Here's how the part is built. I have some questions about the finished solid (model axes, mm). Coordinates: 2 decimals unless noted, no trailing zeros. Loops run counter-clockwise (first coordinate to the right, second up) from the corner with the lowest first, then second, coordinate; pieces in that order, holes last.
from build123d import *

# Parameters (mm, degrees)
SKETCH1_W                 = 12.7
SKETCH1_H                 = 444.5
EXTRUDE1_DEPTH            = 292.1
EXTRUDE1_DEPTH_BACK       = 292.1
CUT_EXTRUDE1_REACH        = 14.7
CUT_EXTRUDE2_REACH        = 14.7
SKETCH5_W                 = 127
SKETCH5_H                 = 43.65625
FILLET2_R                 = 6.35
M6X1_0_TAPPED_HOLE1_D     = 5
M6X1_0_TAPPED_HOLE1_DEPTH = 12.7
SKETCH11_W                = 292.1
SKETCH11_H                = 14.2875
CUT_EXTRUDE3_DEPTH        = 13.7
FILLET3_R                 = 3.175
CUT_EXTRUDE7_DEPTH        = 1
CUT_EXTRUDE7_DEPTH_BACK   = 445.5
CUT_EXTRUDE8_REACH        = 14.7
M6X1_0_TAPPED_HOLE2_D     = 5
M6X1_0_TAPPED_HOLE2_DEPTH = 12.7
M6_CLEARANCE_HOLE1_D      = 6.4
M6_CLEARANCE_HOLE1_DEPTH  = 12.7
CUT_EXTRUDE9_DEPTH        = 13.7
CUT_EXTRUDE10_DEPTH       = 13.7


with BuildPart() as part:
    # Sketch1 → Extrude1 (new body, two sides)
    with BuildSketch(Plane.XY) as extrude1_sk:
        Rectangle(SKETCH1_W, SKETCH1_H)
    extrude(amount=EXTRUDE1_DEPTH)
    extrude(extrude1_sk.sketch, amount=-EXTRUDE1_DEPTH_BACK)

    # Sketch4 → Cut-Extrude1 (cut, up to next)
    with BuildSketch(Plane(origin=(6.35, 0, 0), x_dir=(0, 0, -1), z_dir=(1, 0, 0)), mode=Mode.PRIVATE) as cut_extrude1_sk1:
        Polygon((203.2, 127.79375), (241.3, 127.79375), (241.3, 178.59375), (-241.3, 178.59375), (-241.3, 127.79375), (-203.2, 127.79375), (-203.2, -54.76875), (-241.3, -54.76875), (-241.3, -105.56875), (241.3, -105.56875), (241.3, -54.76875), (203.2, -54.76875), align=None)
    cut_extrude1_tool1 = extrude(cut_extrude1_sk1.sketch, amount=-CUT_EXTRUDE1_REACH, mode=Mode.PRIVATE) & part.part
    add(cut_extrude1_tool1.solids().sort_by_distance((6.35, 36.5125, 0))[0], mode=Mode.SUBTRACT)

    # Sketch5 → Cut-Extrude2 (cut, up to next)
    with BuildSketch(Plane(origin=(6.35, 0, 0), x_dir=(0, 0, -1), z_dir=(1, 0, 0)), mode=Mode.PRIVATE) as cut_extrude2_sk1:
        with Locations((0, 200.421875)):
            Rectangle(SKETCH5_W, SKETCH5_H)
    cut_extrude2_tool1 = extrude(cut_extrude2_sk1.sketch, amount=-CUT_EXTRUDE2_REACH, mode=Mode.PRIVATE) & part.part
    add(cut_extrude2_tool1.solids().sort_by_distance((6.35, 200.421875, 0))[0], mode=Mode.SUBTRACT)

    # Fillet2
    fillet2_edges = [part.edges().sort_by_distance(p)[0] for p in [
        (0, 127.79375, -203.2),
        (0, -54.76875, -203.2),
        (0, -54.76875, -241.3),
        (0, -105.56875, -241.3),
        (0, -105.56875, 241.3),
        (0, -54.76875, 241.3),
        (0, -54.76875, 203.2),
        (0, 127.79375, 203.2),
        (0, 127.79375, 241.3),
        (0, 178.59375, 241.3),
        (0, 178.59375, -241.3),
        (0, 127.79375, -241.3),
    ]]
    fillet(fillet2_edges, radius=FILLET2_R)

    # M6x1.0 Tapped Hole1
    with Locations(Plane(origin=(6.35, 0, 0), x_dir=(0, 0, -1), z_dir=(1, 0, 0))):
        with Locations((101.6, 204.7875), (-101.6, 204.7875), (101.6, -132.23875), (-101.6, -132.23875)):
            Hole(M6X1_0_TAPPED_HOLE1_D / 2, depth=M6X1_0_TAPPED_HOLE1_DEPTH)

    # Sketch11 → Cut-Extrude3 (cut, through all)
    with BuildSketch(Plane(origin=(6.35, 0, 0), x_dir=(0, 0, -1), z_dir=(1, 0, 0))):
        with Locations((0, 185.7375)):
            Rectangle(SKETCH11_W, SKETCH11_H)
    extrude(amount=-CUT_EXTRUDE3_DEPTH, mode=Mode.SUBTRACT)

    # Fillet3
    fillet3_edges = [part.edges().sort_by_distance(p)[0] for p in [
        (0, 192.88125, 63.5),
        (0, 192.88125, -63.5),
        (0, 192.88125, 146.05),
        (0, 178.59375, -146.05),
        (0, 178.59375, 146.05),
        (0, 192.88125, -146.05),
        (0, 222.25, 63.5),
        (0, 222.25, -63.5),
    ]]
    fillet(fillet3_edges, radius=FILLET3_R)

    # Sketch18 → Cut-Extrude7 (cut, two sides)
    with BuildSketch(Plane.XZ.offset(222.25)) as cut_extrude7_sk:
        Polygon((6.35, 1.5875), (6.35, -1.5875), (4.7625, 0), align=None)
    extrude(amount=CUT_EXTRUDE7_DEPTH, mode=Mode.SUBTRACT)
    extrude(cut_extrude7_sk.sketch, amount=-CUT_EXTRUDE7_DEPTH_BACK, mode=Mode.SUBTRACT)

    # Sketch19 → Cut-Extrude8 (cut, up to next)
    with BuildSketch(Plane(origin=(6.35, 0, 0), x_dir=(0, 0, -1), z_dir=(1, 0, 0)), mode=Mode.PRIVATE) as cut_extrude8_sk1:
        with BuildLine():
            Line((104.775, 207.9625), (104.775, 201.6125))
            ThreePointArc((104.775, 201.6125), (101.6, 198.4375), (98.425, 201.6125))
            Line((98.425, 201.6125), (98.425, 207.9625))
            ThreePointArc((98.425, 207.9625), (101.6, 211.1375), (104.775, 207.9625))
        make_face()
    cut_extrude8_tool1 = extrude(cut_extrude8_sk1.sketch, amount=-CUT_EXTRUDE8_REACH, mode=Mode.PRIVATE) & part.part
    add(cut_extrude8_tool1.solids().sort_by_distance((6.35, 204.7875, -101.6))[0], mode=Mode.SUBTRACT)
    # Sketch19 → Cut-Extrude8 (cut, up to next)
    with BuildSketch(Plane(origin=(6.35, 0, 0), x_dir=(0, 0, -1), z_dir=(1, 0, 0)), mode=Mode.PRIVATE) as cut_extrude8_sk2:
        with BuildLine():
            Line((-98.425, 207.9625), (-98.425, 201.6125))
            ThreePointArc((-98.425, 201.6125), (-101.6, 198.4375), (-104.775, 201.6125))
            Line((-104.775, 201.6125), (-104.775, 207.9625))
            ThreePointArc((-104.775, 207.9625), (-101.6, 211.1375), (-98.425, 207.9625))
        make_face()
    cut_extrude8_tool2 = extrude(cut_extrude8_sk2.sketch, amount=-CUT_EXTRUDE8_REACH, mode=Mode.PRIVATE) & part.part
    add(cut_extrude8_tool2.solids().sort_by_distance((6.35, 204.7875, 101.6))[0], mode=Mode.SUBTRACT)
    # Sketch19 → Cut-Extrude8 (cut, up to next)
    with BuildSketch(Plane(origin=(6.35, 0, 0), x_dir=(0, 0, -1), z_dir=(1, 0, 0)), mode=Mode.PRIVATE) as cut_extrude8_sk3:
        with BuildLine():
            Line((-98.425, -129.06375), (-98.425, -135.41375))
            ThreePointArc((-98.425, -135.41375), (-101.6, -138.58875), (-104.775, -135.41375))
            Line((-104.775, -135.41375), (-104.775, -129.06375))
            ThreePointArc((-104.775, -129.06375), (-101.6, -125.88875), (-98.425, -129.06375))
        make_face()
    cut_extrude8_tool3 = extrude(cut_extrude8_sk3.sketch, amount=-CUT_EXTRUDE8_REACH, mode=Mode.PRIVATE) & part.part
    add(cut_extrude8_tool3.solids().sort_by_distance((6.35, -132.23875, 101.6))[0], mode=Mode.SUBTRACT)
    # Sketch19 → Cut-Extrude8 (cut, up to next)
    with BuildSketch(Plane(origin=(6.35, 0, 0), x_dir=(0, 0, -1), z_dir=(1, 0, 0)), mode=Mode.PRIVATE) as cut_extrude8_sk4:
        with BuildLine():
            Line((104.775, -129.06375), (104.775, -135.41375))
            ThreePointArc((104.775, -135.41375), (101.6, -138.58875), (98.425, -135.41375))
            Line((98.425, -135.41375), (98.425, -129.06375))
            ThreePointArc((98.425, -129.06375), (101.6, -125.88875), (104.775, -129.06375))
        make_face()
    cut_extrude8_tool4 = extrude(cut_extrude8_sk4.sketch, amount=-CUT_EXTRUDE8_REACH, mode=Mode.PRIVATE) & part.part
    add(cut_extrude8_tool4.solids().sort_by_distance((6.35, -132.23875, -101.6))[0], mode=Mode.SUBTRACT)

    # M6x1.0 Tapped Hole2
    with Locations(Plane(origin=(6.35, 0, 0), x_dir=(0, 0, -1), z_dir=(1, 0, 0))):
        with Locations((79.375, -191.29375), (-79.375, -191.29375), (250.825, -149.225), (250.825, 193.675), (-250.825, 193.675), (-250.825, -149.225)):
            Hole(M6X1_0_TAPPED_HOLE2_D / 2, depth=M6X1_0_TAPPED_HOLE2_DEPTH)

    # M6 Clearance Hole1
    with Locations(Plane(origin=(6.35, 0, 0), x_dir=(0, 0, -1), z_dir=(1, 0, 0))):
        with Locations((-285.75, -196.85), (-285.75, -66.675), (-285.75, 193.675), (-285.75, 63.5), (285.75, 193.675), (285.75, 63.5), (285.75, -66.675), (285.75, -196.85)):
            Hole(M6_CLEARANCE_HOLE1_D / 2, depth=M6_CLEARANCE_HOLE1_DEPTH)

    # Sketch27 → Cut-Extrude9 (cut, through all)
    with BuildSketch(Plane.ZY.offset(6.35)):
        with BuildLine():
            Line((-209.2325, 33.3375), (-215.5825, 33.3375))
            ThreePointArc((-215.5825, 33.3375), (-218.7575, 36.5125), (-215.5825, 39.6875))
            Line((-215.5825, 39.6875), (-209.2325, 39.6875))
            ThreePointArc((-209.2325, 39.6875), (-206.0575, 36.5125), (-209.2325, 33.3375))
        make_face()
    cut_extrude9 = extrude(amount=-CUT_EXTRUDE9_DEPTH, mode=Mode.SUBTRACT)

    # Mirror1: Cut-Extrude9 across plane
    add(cut_extrude9.mirror(Plane.XY), mode=Mode.SUBTRACT)

    # Sketch29 → Cut-Extrude10 (cut, through all)
    with BuildSketch(Plane(origin=(6.35, 0, 0), x_dir=(0, 0, -1), z_dir=(1, 0, 0))):
        with BuildLine():
            Line((-215.5825, 84.1375), (-209.2325, 84.1375))
            ThreePointArc((-209.2325, 84.1375), (-206.0575, 80.9625), (-209.2325, 77.7875))
            Line((-209.2325, 77.7875), (-215.5825, 77.7875))
            ThreePointArc((-215.5825, 77.7875), (-218.7575, 80.9625), (-215.5825, 84.1375))
        make_face()
        with BuildLine():
            Line((-215.5825, -4.7625), (-209.2325, -4.7625))
            ThreePointArc((-209.2325, -4.7625), (-206.0575, -7.9375), (-209.2325, -11.1125))
            Line((-209.2325, -11.1125), (-215.5825, -11.1125))
            ThreePointArc((-215.5825, -11.1125), (-218.7575, -7.9375), (-215.5825, -4.7625))
        make_face()
    cut_extrude10 = extrude(amount=-CUT_EXTRUDE10_DEPTH, mode=Mode.SUBTRACT)

    # Mirror2: Cut-Extrude10 across plane
    add(cut_extrude10.mirror(Plane.XY), mode=Mode.SUBTRACT)


solid = part.part
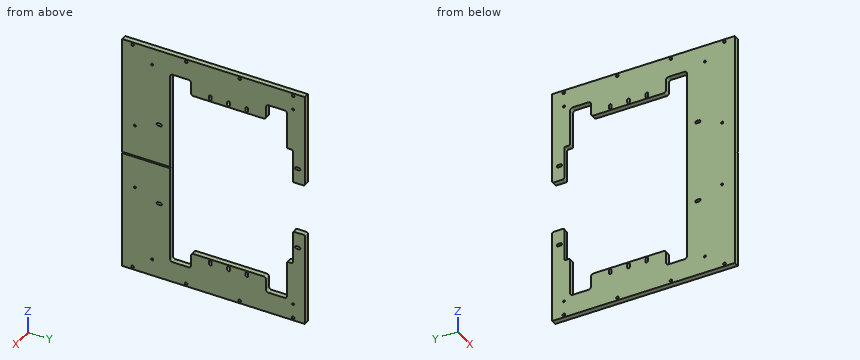
Q1. Suppose I cut it at C-C on x = -1.25. State how many separate pieces and enclosed holes the cut face has, and give its area (3 significant figures).
Q2. Suppose I cut it at B-B on y = -83. Write out the boundary of the cut face in (x, z).
Q3. Suppose I cut it at D-D on z = 52.5. Write out the boundary of the cut face in (x, y).
Q4. Will these pins go through, and if not, where does the flat tip stop? P1, Ø8, axis at y = -149.225, z = -250.825, coming from the +X side; P2, Ø1, axis at x = 4, z = -39.5, coming from the +Y side; P3, Ø5, axis at y = 63.5, z = -285.75, coming from the -X side.
Q5. Suppose I cut it at A-A on z = -113.5. Write out the boundary of the cut face in (x, y).
Q6. Please list where these lines run through material, in increasing order: probe 1 along Y at (x, z) = (-0.75, 285.75) (3 decimals); probe 2 along Y at (x, z) = (-2.5, -229); probe 3 along Z at (x, y) = (3.25, -196.85).
Check values:
1. separate pieces: 1
1. enclosed holes: 24
1. area: 127,000 mm2
2. outline: (-6.35, -292.1) - (6.35, -292.1) - (6.35, -241.3) - (-6.35, -241.3) - close; (-6.35, 241.3) - (6.35, 241.3) - (6.35, 292.1) - (-6.35, 292.1) - close
3. outline: (-6.35, -222.25) - (6.35, -222.25) - (6.35, -105.57) - (-6.35, -105.57) - close
4. P1: stops at x = 6.35
4. P2: stops at y = -105.57
4. P3: passes through
5. outline: (-6.35, -222.25) - (6.35, -222.25) - (6.35, -105.57) - (-6.35, -105.57) - close; (-6.35, 192.88) - (6.35, 192.88) - (6.35, 222.25) - (-6.35, 222.25) - close
6. probe 1: y = -222.25 to -200.05, -193.65 to -69.875, -63.475 to 60.3, 66.7 to 190.475, 196.875 to 222.25
6. probe 2: y = -222.25 to -105.57, -54.77 to 127.79, 178.59 to 222.25
6. probe 3: z = -292.1 to -288.95, -282.55 to 282.55, 288.95 to 292.1
